Autodesk Inventor part; units mm, degrees
ref_plane "YZ Plane" through (0, 0, 0) normal (1, 0, 0) x (0, 1, 0)
ref_plane "XZ Plane" through (0, 0, 0) normal (0, 1, 0) x (-1, 0, 0)
ref_plane "XY Plane" through (0, 0, 0) normal (0, 0, 1) x (1, 0, 0)
sketch "Sketch2" plane through (0, 0, 0) normal (0, 0, 1) x (1, 0, 0)
  line L0 (200, -225) -> (-200, -225)
  line L1 (-200, -225) -> (-200, 225)
  line L2 (-200, 225) -> (200, 225)
  line L3 (200, 225) -> (200, -225)
  line L4 (200, -225) -> (-200, 225) construction
  line L5 (-200, -225) -> (200, 225) construction
  point P0 (0, 0)
  dimension "d0" = 400
  dimension "d1" = 450
extrude "Base" add sketch "Sketch2" along normal blind 360
shell "Shell1" thickness 5 removed faces 1 at (-66.6667, -75, 360)
sketch "Sketch4" plane through (200, -225, 0) normal (1, 0, 0) x (0, 0, -1)
  circle A0 centre (-302.5, 28.75) radius 7.5
  line L0 (-360, 0) -> (-360, 450)
  line L1 (0, 0) -> (-360, 0)
  circle A1 centre (-282.5, 28.75) radius 7.5
  point P0 (0, 225)
  dimension "d18" = 15
  dimension "d19" = 57.5
  dimension "d20" = 28.75
  dimension "d23" = 20
extrude "Cable Holes" cut sketch "Sketch4" against normal up to surface (5 mm away)
sketch "Sketch5" plane through (-195, 220, 5) normal (0, 0, 1) x (1, 0, 0)
  line L0 (349.75, -399.75) -> (40.25, -399.75) construction
  line L1 (40.25, -399.75) -> (40.25, -40.25) construction
  line L2 (40.25, -40.25) -> (349.75, -40.25) construction
  line L3 (349.75, -40.25) -> (349.75, -399.75) construction
  line L4 (349.75, -399.75) -> (40.25, -40.25) construction
  line L5 (40.25, -399.75) -> (349.75, -40.25) construction
  circle A0 centre (40.25, -40.25) radius 2.75
  circle A1 centre (349.75, -40.25) radius 2.75
  circle A2 centre (40.25, -399.75) radius 2.75
  circle A3 centre (349.75, -399.75) radius 2.75
  point P0 (195, -220)
  dimension "d30" = 309.5
  dimension "d31" = 359.5
  dimension "d32" = 5.5
  dimension "d35" = 309.5
  dimension "d38" = 359.5
extrude "Mount Holes inner walls" cut sketch "Sketch5" against normal up to surface (5 mm away)
sketch "Sketch6" plane through (200, -225, 0) normal (1, 0, 0) x (0, 0, -1)
  circle A0 centre (-314.25, 404.75) radius 2.625
  line L0 (-360, 445) -> (-360, 5) construction
  line L1 (-360, 445) -> (-360, 155) construction
  line L2 (-314.25, 404.75) -> (-314.25, 45.25) construction
  circle A1 centre (-314.25, 45.25) radius 2.625
  line L3 (-5, 5) -> (-5, 445)
  point P0 (0, 225)
  point P1 (-314.25, 225)
  point P2 (-360, 225)
  dimension "d43" = 5.25
  dimension "d44" = 359.5
  dimension "d46" = 5.25
  dimension "d63" = 309.25
extrude "Extrusion5" cut sketch "Sketch6" against normal up to surface (5 mm away)
mirror "Mirror2" about plane through (0, 0, 0) normal (1, 0, 0) of "Extrusion5"
sketch "Sketch7" plane through (0, 0, 0) normal (0, 0, -1) x (-1, 0, 0)
  circle A0 centre (-113.0307, -138.0307) radius 19
  circle A1 centre (-129.0307, -122.0307) radius 2.15
  line L0 (-30.7163, 0) -> (40.9179, 0) construction
  line L1 (0, 50.4838) -> (0, -80.5394) construction
  circle A2 centre (-97.0307, -122.0307) radius 2.15
  circle A3 centre (-129.0307, -154.0307) radius 2.15
  circle A4 centre (-97.0307, -154.0307) radius 2.15
  circle A5 centre (-154.75, -179.75) radius 2.75 construction
  line L2 (-154.75, -179.75) -> (-113.0307, -138.0307) construction
  line L3 (-154.75, -179.75) -> (-95.75, -179.75) construction
  line L4 (-129.0307, -122.0307) -> (-97.0307, -122.0307) construction
  line L5 (-129.0307, -154.0307) -> (-129.0307, -122.0307) construction
  point P0 (0, 0)
  point P1 (-113.0307, -122.0307)
  point P2 (-129.0307, -138.0307)
  dimension "d49" = 4.3
  dimension "d52" = 32
  dimension "d55" = 32
  dimension "d58" = 38
  dimension "d59" = 59
  dimension "d60" = 45
extrude "Fan holes" cut sketch "Sketch7" against normal up to surface (5 mm away)
equation "\"d20\" = 0.5 * d19"
equation "\"d35\" = d30"
equation "\"d38\" = d31"
equation "\"d44\" = d31"
equation "\"d46\" = d43"
equation "\"d55\" = d52"
properties part number "mouse_SP_shell"
Work out the finished part from the listing and answer in its coordinate system (mm). A direction names the side the tool comes from. Give positions to 0.01 mm unless a question says otherwise; leave off trailing zeros. Loops run counter-clockwise (first coordinate to the right, second up) from the corner with the lowest first, then second, coordinate; pieces in that order, holes last. Notation, with made-up numbers: (77.25, 40.5) -> (110.25, 40.5) arc R33 ccw to (110.25, 77.5) -> close; hole circle Ø5 at (-2.75, 50.25). An arc over 180 degrees is marked (long way). One line per question, with ' | ' between items. Start each with the question number.
1) Section D-D, the plane y = -105 is taken. Determine the outline of the cut face in (x, z).
2) Section A-A, the plane x = 36 is taken. Determine the outline of the cut face in (y, z), then the cut area to 3 significant figures.
3) For faces 1 (the face through (3, -220, 180)), 2 (the face through (197.535, -191.181, 308.028)), 3 (the face through (-200, -3, 177)), determine the directions among +Z, -Z, +X, -X, +Y, -Y from which every point of the face is accessible in a straight line to the end or side of a thin tool.
4) This flat-tipped pin is pushed along its axis until it touches: pin 1 (10 mm diameter, centred on x = 143.5, y = -39.5, fed in from +Z). Where does it stop, or does it pass through?
5) Section B-B, the plane z = 328 is taken. Determine the outline of the cut face in (x, y).
6) Section C-C, the plane x = 114.5 is taken. Determine the outline of the cut face in (y, z).
7) Determine the mould class of faces 4 (the face through (-3, 3, 0)), 5 (the face through (195, 3, 180)), 6 (the face through (-3, 225, 177)) for opening direction Y: +Y half, -Y half, draft (parallel to the pull), parting line (faces both ways), or undercut.
8) Straight lines are drawn through the part: L1, parallel to X at y = -179.75, z = 2.3; L2, parallel to Y at x = 154, z = 3; L3, parallel to Z at x = -196.1, y = 179.75 (3 decimals). For each, find the intervals that lie inside material, in ascending order.
Resolved:
1) outline: (-200, 0) -> (200, 0) -> (200, 360) -> (195, 360) -> (195, 5) -> (-195, 5) -> (-195, 360) -> (-200, 360) -> close
2) outline: (-225, 0) -> (225, 0) -> (225, 360) -> (220, 360) -> (220, 5) -> (-220, 5) -> (-220, 360) -> (-225, 360) -> close | area: 5,800 mm2
3) face 1: +Z | face 2: +X | face 3: +Z, -Z, -X, +Y, -Y
4) pin 1: z = 5
5) outline: (-200, -225) -> (200, -225) -> (200, 225) -> (-200, 225) -> close; hole (-195, -220) -> (195, -220) -> (195, 220) -> (-195, 220) -> close
6) outline: (-225, 0) -> (-156.97, 0) -> (-156.97, 5) -> (-220, 5) -> (-220, 360) -> (-225, 360) -> close; (-119.09, 0) -> (225, 0) -> (225, 360) -> (220, 360) -> (220, 5) -> (-119.09, 5) -> close
7) face 4: draft | face 5: undercut | face 6: +Y half
8) L1: -200 to -157.5, -152 to 152, 157.5 to 200 | L2: -225 to -182.4, -177.1 to 177.1, 182.4 to 225 | L3: 0 to 311.625, 316.875 to 360
